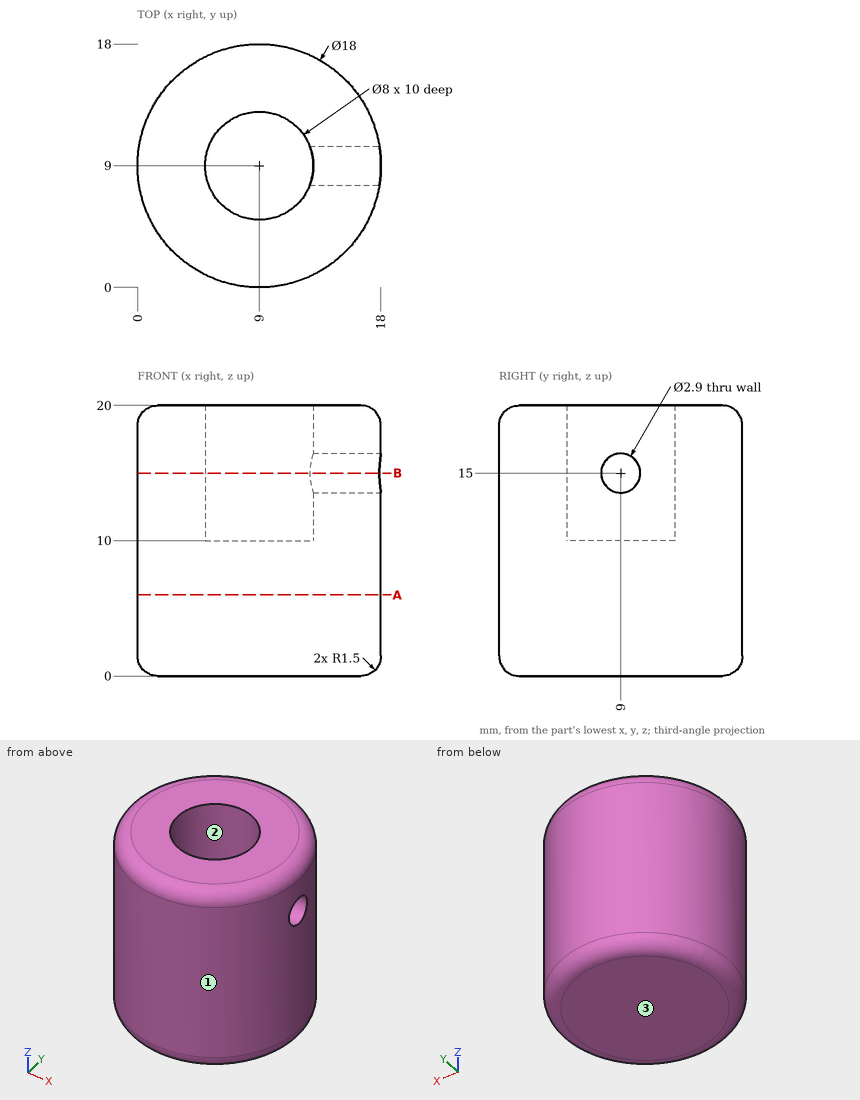
Could you check a few things on this drawing? It's one solid part, dimensions in mm from its lowest x, y, z. Round coordinates to 2 decimals unless told otherwise and drop trailing zeros. Loops run counter-clockwise (first coordinate to the right, second up) from the corner with the lowest first, then second, coordinate; pieces in that order, holes last. Notation, with made-up numbers: M -35,-32 L 14,-32 A15 cw 14,-28 Z; hole C -20.5,18 d3. An arc over 180 degrees is marked long. Write item = value, one per line. Start each with the question number.
(1) Suppose I cut it at B-B on z = 15. Write out the boundary of the cut face in (x, y).
(2) I need wall thicknesses on line 1 along Y through (x, z) = (9, 17); line 2 along Z through (x, y) = (7.5, 12.5); line 3 along Y through (x, z) = (9, 6.5). Which ranges of each line are inside material? Lowest first, please.
(3) I'm going to push flat-ended pins straight in: P1, Ø5, axis at y = 16, z = 14, coming from the +X side; P2, Ø7, axis at x = 9, y = 9, coming from the +Z side; P3, Ø6, axis at x = 4.5, z = 12, coming from the -Y side. Where does each tip first touch, or does it pass through?
(4) If we mould it in two halves opening along Y, with no side actions, what happens to the marked faces 1, 2 and 3? For each: released by +Y, released by -Y, zero draft, split by the parting line, or undercut.
(5) Suppose I cut it at A-A on z = 6. Write out the boundary of the cut face in (x, y).
Answer block:
q1.outline = M 12.73,7.55 A4 cw long 12.73,10.45 L 17.88,10.45 A9 ccw long 17.88,7.55 Z
q2.line_1 = 0 to 5, 13 to 18
q2.line_2 = 0 to 10
q2.line_3 = 0 to 18
q3.P1 = 16.79
q3.P2 = 10
q3.P3 = 0.13
q4.face_1 = split by the parting line
q4.face_2 = undercut
q4.face_3 = zero draft
q5.outline = C 9,9 d18
